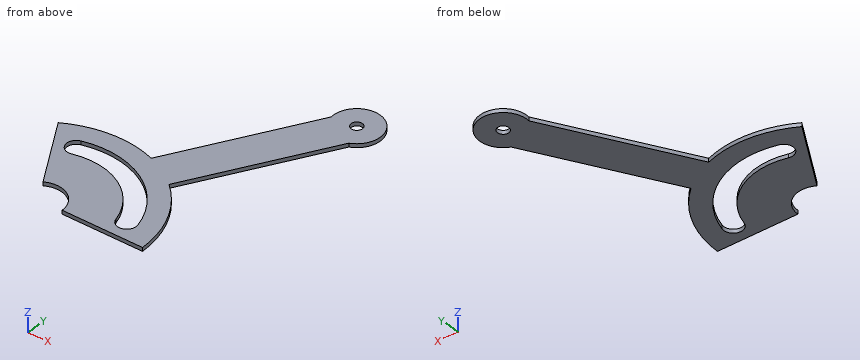
```python
from build123d import *

# Parameters (mm, degrees)
BASE_FLANGE1_DEPTH = 2
CUT_EXTRUDE1_DEPTH = 10
SKETCH9_R          = 3
CUT_EXTRUDE2_DEPTH = 10


# Sheet-metal steps are written as plain solids
with BuildPart() as part:
    # Sketch1 → Base-Flange1 (new body)
    with BuildSketch(Plane.XY):
        with BuildLine():
            Line((12.5, 0), (55, 0))
            ThreePointArc((55, 0), (49.942986861, 23.036884846), (35.701888604, 41.837484988))
            Line((35.701888604, 41.837484988), (75.701888604, 111.119517291))
            ThreePointArc((75.701888604, 111.119517291), (77.041634566, 133.440025366), (58.381380528, 121.119517291))
            Line((58.381380528, 121.119517291), (18.381380528, 51.837484988))
            ThreePointArc((18.381380528, 51.837484988), (-5.02096593, 54.770337785), (-27.5, 47.631397208))
            Line((-27.5, 47.631397208), (-6.25, 10.825317547))
            ThreePointArc((-6.25, 10.825317547), (6.25, 10.825317547), (12.5, 0))
        make_face()
    extrude(amount=-BASE_FLANGE1_DEPTH)

    # Sketch6 → Cut-Extrude1 (cut)
    with BuildSketch(Plane(origin=(0, 0, -2), x_dir=(-1, 0, 0), z_dir=(0, 0, -1))):
        with BuildLine():
            ThreePointArc((12.04274553, 43.35864712), (-22.5, 38.97114317), (-43.571062645, 11.25))
            ThreePointArc((-43.571062645, 11.25), (-39.979833462, 5.158770817), (-33.888604279, 8.75))
            ThreePointArc((-33.888604279, 8.75), (-17.5, 30.310889132), (9.366579857, 33.723392205))
            ThreePointArc((9.366579857, 33.723392205), (15.522290151, 37.202936826), (12.04274553, 43.35864712))
        make_face()
    extrude(amount=-CUT_EXTRUDE1_DEPTH, mode=Mode.SUBTRACT)

    # Sketch9 → Cut-Extrude2 (cut)
    with BuildSketch(Plane(origin=(0, 0, -2), x_dir=(-1, 0, 0), z_dir=(0, 0, -1))):
        with Locations((-70.791634566, 122.614707819)):
            Circle(SKETCH9_R)
    extrude(amount=-CUT_EXTRUDE2_DEPTH, mode=Mode.SUBTRACT)


solid = part.part
```
Geometry check sheet. Reference: the model listing, model coordinates, mm. Coordinates: 2 decimals unless noted, no trailing zeros. Order: outer loops, then holes, each group sorted by start corner. A loop starts at its lowest first (then second) coordinate and runs counter-clockwise, first axis right, second up. Notation, with made-up numbers: (35, -16) - (41, -16) arc R5 ccw to (41, -10) - close; hole circle Ø9 at (17, 76.5). An arc over 180 degrees is marked (long way). Use one line per item in the form item = value.
1. Scan lines: line 1 (Y direction, x = 40, z = -1); line 2 (Y direction, x = 13, z = -1.7); line 3 (Y direction, x = 16, z = -1.2). Record each from-to range of solid material in increasing order.
Here are the results:
line_1 = 0 to 5.16, 20.62 to 37.75, 49.28 to 89.28
line_2 = 0 to 32.5, 43.08 to 53.44
line_3 = 0 to 31.13, 42.06 to 52.62
2. Section check A-A (y = 20). Record the boundary of the cut face in (x, z).
Here are the results:
outline = (-11.55, -2) - (28.72, -2) - (28.72, 0) - (-11.55, 0) - close; (40.31, -2) - (51.23, -2) - (51.23, 0) - (40.31, 0) - close
3. Gauge pin test, flat end, axial feed: pin 1 (5.5 mm diameter, centred on x = 70.79, y = 122.61, fed in from +Z). Record the tip position at first contact, or that the pin passes through.
Here are the results:
pin_1 = through
4. Section check B-B (x = 22). Record the boundary of the cut face in (y, z).
Here are the results:
outline = (0, -2) - (27.22, -2) - (27.22, 0) - (0, 0) - close; (39.26, -2) - (58.11, -2) - (58.11, 0) - (39.26, 0) - close
5. Section check C-C (z = -1.65). Record the boundary of the cut face in (x, y), then the cut area to 3 significant figures.
Here are the results:
outline = (-27.5, 47.63) - (-6.25, 10.83) arc R12.5 cw to (12.5, 0) - (55, 0) arc R55 ccw to (35.7, 41.84) - (75.7, 111.12) arc R12.5 ccw (long way) to (58.38, 121.12) - (18.38, 51.84) arc R55 ccw to start; hole (-12.04, 43.36) arc R5 ccw to (-9.37, 33.72) arc R35 cw to (33.89, 8.75) arc R5 ccw to (43.57, 11.25) arc R45 ccw to start; hole circle Ø6 at (70.79, 122.61)
area = 4,270 mm²
6. Section check D-D (y = 117). Record the boundary of the cut face in (x, z).
Here are the results:
outline = (56, -2) - (81.96, -2) - (81.96, 0) - (56, 0) - close
